```python
from build123d import *

# Parameters (mm, degrees)
SKETCH2_W                  = 58.42
SKETCH2_H                  = 23
TWOLEGS_DEPTH              = 14.5
LEGSLOTS_DEPTH             = 62.281289151
SKETCH6_W                  = 3.81
SKETCH6_H                  = 2.54
GROOVE_DEPTH               = 25.4
MIDDLEBRIDGECUT_DEPTH      = 25.4
SKETCH8_W                  = 17
SKETCH8_H                  = 14.5
BRIDGE_DEPTH               = 17
BRIDGEUNDERCUT_REACH       = 53.567
SKETCH15_W                 = 17
SKETCH15_H                 = 8.4
MIRROR14_START             = 10.281893146
MIRROR14_OUTLINE_W         = 6.1
MIRROR14_OUTLINE_H         = 17
MIRROR14_DEPTH             = 17
CLAMPINCLINE_DEPTH         = 17
EXTRUDECONNECTOR_DEPTH     = 35.56
CONNECTORDRAFT_REACH       = 111.361
CONNECTORGROOVE_REACH      = 94.034
CONNECTORHOLE_REACH        = 111.361
SKETCH25_R                 = 2.4765
SKETCH26_R                 = 3.15
BRIDGEHOLE_DEPTH           = 4.5
FILLET1_R                  = 15.24
FILLET2_R                  = 5.08
CONNECTORDRAFT2_DEPTH      = 93.034308057
CONNECTORDRAFT2_DEPTH_BACK = 93.034308057
LEGSHORTEN_REACH           = 98.848
SKETCH28_W                 = 6.35
SKETCH28_H                 = 23


with BuildPart() as part:
    # Sketch2 → twolegs (new body)
    with BuildSketch(Plane(origin=(0, 0, 0), x_dir=(1, 0, 0), z_dir=(0, 1, 0))):
        Rectangle(SKETCH2_W, SKETCH2_H)
    twolegs = extrude(amount=TWOLEGS_DEPTH)

    # Sketch4 → legslots (cut, symmetric)
    with BuildSketch(Plane.ZY.offset(29.21)):
        with BuildLine():
            Line((-8.2, -58.921978701), (-8.2, 0))
            ThreePointArc((-8.2, 0), (0, 8.2), (8.2, 0))
            Line((8.2, 0), (8.2, -58.921978701))
            Line((8.2, -58.921978701), (8.2, -176.765936102))
            Line((8.2, -176.765936102), (-8.2, -176.765936102))
            Line((-8.2, -176.765936102), (-8.2, -58.921978701))
        make_face()
    legslots = extrude(amount=LEGSLOTS_DEPTH, both=True, mode=Mode.SUBTRACT)

    # Sketch6 → groove (cut)
    with BuildSketch(Plane(origin=(0, 0, -11.5), x_dir=(-1, 0, 0), z_dir=(0, 0, -1))):
        with Locations((14.605, 13.23)):
            Rectangle(SKETCH6_W, SKETCH6_H)
    groove = extrude(amount=-GROOVE_DEPTH, mode=Mode.SUBTRACT)

    # Sketch7 → middlebridgecut (cut)
    with BuildSketch(Plane(origin=(0, 14.5, 0), x_dir=(1, 0, 0), z_dir=(0, 1, 0))):
        Polygon((12.468268199, 11.5), (29.21, 8.54798098), (29.21, 11.5), align=None)
    extrude(amount=-MIDDLEBRIDGECUT_DEPTH, mode=Mode.SUBTRACT)

    # Sketch8 → bridge (add)
    with BuildSketch(Plane(origin=(2.342580113, 0, -13.285432008), x_dir=(-0.9848077530122094, 0, -0.17364817766692317), z_dir=(0.17364817766692317, 0, -0.9848077530122094))):
        with Locations((-18.781893146, 7.25)):
            Rectangle(SKETCH8_W, SKETCH8_H)
    extrude(amount=BRIDGE_DEPTH)

    # Sketch15 → bridgeundercut (cut, up to next)
    with BuildSketch(Plane(origin=(10.125688085, 0, 1.785432008), x_dir=(-0.17364817766692317, 0, 0.9848077530122095), z_dir=(-0.9848077530122095, 0, -0.17364817766692317)), mode=Mode.PRIVATE) as bridgeundercut_sk1:
        with Locations((-21.990381211, 4.2)):
            Rectangle(SKETCH15_W, SKETCH15_H)
    bridgeundercut_tool1 = extrude(bridgeundercut_sk1.sketch, amount=-BRIDGEUNDERCUT_REACH, mode=Mode.PRIVATE) & part.part
    bridgeundercut = bridgeundercut_tool1.solids().sort_by_distance((13.944278, 4.2, -19.870866))[0]
    add(bridgeundercut, mode=Mode.SUBTRACT)

    # Mirror14: read off the stored shape, not the designer's step
    # Mirror14 outline → Mirror14 (add)
    with BuildSketch(Plane(origin=(0, 0, 0), x_dir=(0, 1, 0), z_dir=(0.9848077530122094, 0, 0.17364817766692306)).offset(MIRROR14_START)):
        with Locations((11.45, -38.990381211)):
            Rectangle(MIRROR14_OUTLINE_W, MIRROR14_OUTLINE_H)
    extrude(amount=MIRROR14_DEPTH)

    # Mirror15: twolegs across plane
    add(twolegs.mirror(Plane(origin=(5.294599134, 0, -30.027163809), x_dir=(0.9848077530122092, 0, 0.17364817766692314), z_dir=(0.17364817766692314, 0, -0.9848077530122094))))

    # Mirror16: legslots, groove, bridgeundercut across plane
    add(legslots.mirror(Plane(origin=(5.294599134, 0, -30.027163809), x_dir=(0.9848077530122092, 0, 0.17364817766692314), z_dir=(0.17364817766692314, 0, -0.9848077530122094))), mode=Mode.SUBTRACT)
    add(groove.mirror(Plane(origin=(5.294599134, 0, -30.027163809), x_dir=(0.9848077530122092, 0, 0.17364817766692314), z_dir=(0.17364817766692314, 0, -0.9848077530122094))), mode=Mode.SUBTRACT)
    add(bridgeundercut.mirror(Plane(origin=(5.294599134, 0, -30.027163809), x_dir=(0.9848077530122092, 0, 0.17364817766692314), z_dir=(0.17364817766692314, 0, -0.9848077530122094))), mode=Mode.SUBTRACT)

    # Sketch21 → clampincline (cut, symmetric)
    with BuildSketch(Plane(origin=(5.294599134, 0, -30.027163809), x_dir=(-0.9848077530122094, 0, -0.17364817766692314), z_dir=(0.17364817766692314, 0, -0.9848077530122094))):
        Polygon((-24.800533146, 14.5), (-10.281893146, 9.782607901), (-10.281893146, 14.5), align=None)
    extrude(amount=CLAMPINCLINE_DEPTH, both=True, mode=Mode.SUBTRACT)

    # Sketch22 → extrudeconnector (add)
    with BuildSketch(Plane(origin=(-1.864440892, 5.826679393, -0.328751233), x_dir=(-0.19370062592752282, -0.006629130978421877, 0.98103828780418), z_dir=(-0.30432233187297286, 0.9510565162951554, -0.05366023794131847))):
        Polygon((-48.081564355, 27.0422172), (-14.089388689, 27.771596028), (-13.761901853, 12.509307601), (-47.754077519, 11.779928772), align=None)
    extrude(amount=EXTRUDECONNECTOR_DEPTH)

    # Sketch23 → connectordraft (cut, up to next)
    with BuildSketch(Plane(origin=(26.288198213, 8.673320607, 4.635318619), x_dir=(0.3484357800023436, -0.8710369750422688, -0.34624715930007605), z_dir=(0.9366078308002519, 0.30901699437494146, 0.16514923091290587)), mode=Mode.PRIVATE) as connectordraft_sk1:
        Polygon((-21.922562345, 53.820435592), (-0.501791973, 52.073152935), (-19.112117469, 60.231472918), align=None)
    connectordraft_tool1 = extrude(connectordraft_sk1.sketch, amount=-CONNECTORDRAFT_REACH, mode=Mode.PRIVATE) & part.part
    # Sketch23 → connectordraft (cut, up to next)
    with BuildSketch(Plane(origin=(26.288198213, 8.673320607, 4.635318619), x_dir=(0.3484357800023436, -0.8710369750422688, -0.34624715930007605), z_dir=(0.9366078308002519, 0.30901699437494146, 0.16514923091290587)), mode=Mode.PRIVATE) as connectordraft_sk2:
        Polygon((-14.152524229, 20.933828779), (-32.762849725, 29.092148762), (-29.952404848, 35.503186089), align=None)
    connectordraft_tool2 = extrude(connectordraft_sk2.sketch, amount=-CONNECTORDRAFT_REACH, mode=Mode.PRIVATE) & part.part
    add(connectordraft_tool1.solids().sort_by_distance((23.504771, 41.877747, -41.709143))[0], mode=Mode.SUBTRACT)
    add(connectordraft_tool2.solids().sort_by_distance((18.411091, 41.877747, -12.821449))[0], mode=Mode.SUBTRACT)

    # connectorgroove: up to this plane
    connectorgroove_end = Plane(origin=(-43.786464147, 27.065475321, -48.835745626), z_dir=(-0.06506049659943954, -0.3097627963249175, 0.9485853371179643))
    # Sketch24 → connectorgroove (cut, up to the surface)
    with BuildSketch(Plane(origin=(2.342580113, 0, -13.285432008), x_dir=(-0.9848077530122095, 0, -0.1736481776669232), z_dir=(0.1736481776669232, 0, -0.9848077530122095)), mode=Mode.PRIVATE) as connectorgroove_sk1:
        Polygon((-9.788420854, 30.987981431), (-12.735554786, 31.945563293), (-8.026135792, 46.439664601), (-5.079001859, 45.482082739), align=None)
    connectorgroove_tool1 = split(extrude(connectorgroove_sk1.sketch, amount=CONNECTORGROOVE_REACH, mode=Mode.PRIVATE), bisect_by=connectorgroove_end, keep=Keep.BOTH, mode=Mode.PRIVATE)
    add(connectorgroove_tool1.solids().sort_by_distance((11.114537, 38.713823, -11.738699))[0], mode=Mode.SUBTRACT)

    # connectorhole: up to this face of the body (flat: up to its plane)
    connectorhole_end = Plane(part.part.faces().sort_by_distance((10.456046087, 25.296664487, -29.117061452))[0])
    # Sketch25 → connectorhole (cut, up to the picked face)
    with BuildSketch(Plane(origin=(26.288198213, 8.673320607, 4.635318619), x_dir=(0.3484357800023436, -0.8710369750422688, -0.34624715930007605), z_dir=(0.9366078308002519, 0.30901699437494146, 0.16514923091290587)), mode=Mode.PRIVATE) as connectorhole_sk1:
        with Locations(Location((-18.958611536, 41.602440846, 0), (0, 0, 159.447358614))):
            Circle(SKETCH25_R)
    connectorhole_tool1 = split(extrude(connectorhole_sk1.sketch, amount=-CONNECTORHOLE_REACH, mode=Mode.PRIVATE), bisect_by=connectorhole_end, keep=Keep.BOTH, mode=Mode.PRIVATE)
    add(connectorhole_tool1.solids().sort_by(Axis((21.215591, 41.072519, -27.219863), (-0.9366078308002519, -0.30901699437494146, -0.16514923091290587)))[0], mode=Mode.SUBTRACT)

    # Sketch26 → bridgehole (cut)
    with BuildSketch(Plane.XZ.offset(-8.4)):
        with Locations(Location((24.012358933, -26.726717738, 0), (0, 0, 270))):
            Circle(SKETCH26_R)
    extrude(amount=-BRIDGEHOLE_DEPTH, mode=Mode.SUBTRACT)

    # Fillet1
    fillet1_edges = [part.edges().sort_by_distance(p)[0] for p in [
        (29.21, 11.45, -8.54798098),
        (35.114038041, 11.45, -42.031444582),
    ]]
    fillet(fillet1_edges, radius=FILLET1_R)

    # Fillet2
    # the kernel refuses this fillet: 5.08 mm, written as the material it adds along each edge
    with BuildSketch(Plane(origin=(-25.052907191, 14.5, -18.115995569), x_dir=(-0.17364817766692314, 0, 0.9848077530122094), z_dir=(0.9848077530122094, 0, 0.17364817766692314))) as fillet2_piece_1_section:
        with BuildLine():
            CenterArc((FILLET2_R, -FILLET2_R), FILLET2_R, 90, 90)
            Line((0, -FILLET2_R), (0, 0))
            Line((0, 0), (FILLET2_R, 0))
        make_face()
    fillet2_piece_1 = extrude(amount=65.31864, mode=Mode.PRIVATE)
    fillet2_piece_1 = split(fillet2_piece_1, bisect_by=Plane(origin=(-12.7, 14.5, -18.115995569), z_dir=(1, 0, 0)), keep=Keep.TOP, mode=Mode.PRIVATE)
    fillet2_piece_1 = split(fillet2_piece_1, bisect_by=Plane(origin=(-25.052907191, 14.5, -11.5), z_dir=(0, 0, 1)), keep=Keep.TOP, mode=Mode.PRIVATE)
    fillet2_piece_1 = split(fillet2_piece_1, bisect_by=Plane(origin=(21.81803989, 29.964230294, -9.851382987), z_dir=(-0.9366078308002517, -0.30901699437494173, -0.16514923091290615)), keep=Keep.TOP, mode=Mode.PRIVATE)
    add(fillet2_piece_1)
    with BuildSketch(Plane(origin=(-19.14886915, 14.5, -51.599459172), x_dir=(0.17364817766692314, 0, -0.9848077530122094), z_dir=(0.9848077530122094, 0, 0.17364817766692314))) as fillet2_piece_2_section:
        with BuildLine():
            CenterArc((FILLET2_R, FILLET2_R), FILLET2_R, 180, 90)
            Line((0, FILLET2_R), (0, 0))
            Line((0, 0), (FILLET2_R, 0))
        make_face()
    fillet2_piece_2 = extrude(amount=65.31864, mode=Mode.PRIVATE)
    fillet2_piece_2 = split(fillet2_piece_2, bisect_by=Plane(origin=(27.722077931, 29.964230294, -43.33484659), z_dir=(-0.9366078308002517, -0.30901699437494173, -0.16514923091290615)), keep=Keep.TOP, mode=Mode.PRIVATE)
    fillet2_piece_2 = split(fillet2_piece_2, bisect_by=Plane(origin=(-7.540933418, 14.5, -47.374516084), z_dir=(0.9396926207859135, 0, 0.342020143325655)), keep=Keep.TOP, mode=Mode.PRIVATE)
    fillet2_piece_2 = split(fillet2_piece_2, bisect_by=Plane(origin=(-16.886065398, 14.5, -57.816461387), z_dir=(0.342020143325655, 0, -0.9396926207859134)), keep=Keep.TOP, mode=Mode.PRIVATE)
    add(fillet2_piece_2)

    # Sketch27 → connectordraft2 (cut, two sides: drawn at the far end of the back side and taken through both)
    with BuildSketch(Plane(origin=(2.342580113, 0, -13.285432008), x_dir=(-0.9848077530122095, 0, -0.1736481776669232), z_dir=(0.1736481776669232, 0, -0.9848077530122095)).offset(-CONNECTORDRAFT2_DEPTH_BACK)):
        Polygon((-10.919012309, 47.37961716), (-20.091114151, 28.994101308), (-13.811888826, 48.319569719), align=None)
        Polygon((-2.186125342, 44.54213018), (-5.572474151, 24.27670921), (0.706751174, 43.602177621), align=None)
    extrude(amount=CONNECTORDRAFT2_DEPTH + CONNECTORDRAFT2_DEPTH_BACK, mode=Mode.SUBTRACT)

    # legshorten: up to this face of the body (flat: up to its plane)
    legshorten_end = Plane(part.part.faces().sort_by_distance((-3.474076782, 0, -9.752083384))[0])
    # Sketch28 → legshorten (cut, up to the picked face)
    with BuildSketch(Plane(origin=(0, 14.5, 0), x_dir=(1, 0, 0), z_dir=(0, 1, 0)), mode=Mode.PRIVATE) as legshorten_sk1:
        with Locations((-26.035, 0)):
            Rectangle(SKETCH28_W, SKETCH28_H)
    legshorten_tool1 = split(extrude(legshorten_sk1.sketch, amount=-LEGSHORTEN_REACH, mode=Mode.PRIVATE), bisect_by=legshorten_end, keep=Keep.BOTH, mode=Mode.PRIVATE)
    legshorten = legshorten_tool1.solids().sort_by(Axis((-26.035, 14.5, 0), (0, -1, 0)))[0]
    add(legshorten, mode=Mode.SUBTRACT)

    # Mirror17: legshorten across plane
    add(legshorten.mirror(Plane(origin=(5.294599134, 0, -30.027163809), x_dir=(0.9848077530122092, 0, 0.17364817766692314), z_dir=(0.17364817766692314, 0, -0.9848077530122094))), mode=Mode.SUBTRACT)


solid = part.part
```
Work out the finished part from the listing and answer in its coordinate system (mm). A direction names the side the tool comes from. Round coordinates to 2 decimals unless told otherwise and drop trailing zeros. Loops run counter-clockwise (first coordinate to the right, second up) from the corner with the lowest first, then second, coordinate; pieces in that order, holes last. Notation, with made-up numbers: M 67.5,-40 L 88.5,-40 A17 cw 88.5,-29 Z; hole C 6,62.25 d5. An arc over 180 degrees is marked long. Use CSV: the item, a comma, the result in double quotes.
Q1. The mould has two halves that part along Y. Classify faces 1 (the flat face through (-1.29, 13.24, -64.55)), 2 (the flat face through (14.619, 46.916, -28.24)), 3 (the cylindrical face through (18.453, 37.556, -27.733)): pulls with the +Y half, pulls with the -Y half, needs draft (parallel to the pull), parting line crosses it, or undercut.
Determined:
face 1,"needs draft"
face 2,"pulls with the +Y half"
face 3,"undercut"
Q2. Each of these flat-tipped pins is pushed along its axis until it touches: pin 1 (7 mm diameter, centred on x = 24.5, z = -25, fed in from -Y); pin 2 (2 mm diameter, centred on x = 22, z = -16, fed in from +Y); pin 3 (5.5 mm diameter, centred on x = 24.01, z = -26.73, fed in from -Y). Where does it stop, or does it pass through?
Determined:
pin 1,"y = 8.4"
pin 2,"y = 33.41"
pin 3,"y = 12.9"
Q3. Section C-C, the plane y = 28 is taken. Determine the outline of the cut face in (x, z), then the cut area to 3 significant figures.
Determined:
outline,"M 7.44,-13.69 L 12.9,-44.64 L 25.02,-43.81 L 28.35,-43.22 L 22.45,-9.74 L 19.12,-10.33 Z"
area,"510 mm2"
Q4. Section B-B, the plane z = 0 is taken. Determine the outline of the cut face in (x, y).
Determined:
outline,"M -22.86,8.2 L 29.21,8.2 L 29.21,14.5 L -12.7,14.5 L -12.7,11.96 L -16.51,11.96 L -16.51,14.5 L -22.86,14.5 Z"
Q5. Section A-A, the plane y = 3.5 is taken. Determine the outline of the cut face in (x, z).
Determined:
outline,"M -22.86,-11.5 L 12.47,-11.5 L 29.21,-8.55 L 29.21,-7.42 L -22.86,-7.42 Z; M -22.86,7.42 L 29.21,7.42 L 29.21,11.5 L -22.86,11.5 Z; M -14.83,-57.07 L -13.43,-60.9 L 35.5,-43.1 L 35.11,-42.03 L 18.37,-44.98 Z; M -8.36,-74.84 L -6.96,-78.68 L 41.97,-60.87 L 40.57,-57.03 Z"
Q6. Section D-D, the plane y = 21.5 is taken. Determine the outline of the cut face in (x, z).
Determined:
outline,"M 8.72,-12.16 L 14.62,-45.64 L 30.43,-42.86 L 24.53,-9.37 Z"
Q7. A tool of negligible diameter and unlimited length cuts with its end or side. For faces 4 (the flat face through (15.38, 9.08, -28.01)), 5 (the flat face through (20.722, 4.141, -10.045)), 6 (the flat face through (-16.51, 13, 0)), 7 (the flat face through (24, 12.9, -27)), from which of +Z, -Z, +X, -X, +Y, -Y can it reach the whole face along a straight path? Write none if from no direction.
Determined:
face 4,"-X, -Y"
face 5,"+X, -Y"
face 6,"+Z, -Z, +Y"
face 7,"-Y"
Q8. Consider L1, parallel to Y at x = 18.5, z = 2.5; L2, parallel to Y at x = 22, z = -65.5; L3, parallel to X at y = 41, z = -39.5. Determine where each line is inside the solid, lowest interval first.
Determined:
L1,"7.81 to 14.5"
L2,"0 to 14.5"
L3,"9.79 to 13.6, 16.91 to 21.28"
